from build123d import *

# Parameters (mm, degrees)
SKETCH_1_W          = 30
SKETCH_1_H          = 65
EXTRUDE_1_DEPTH     = 3
SKETCH_2_R          = 1.505
CUT_EXTRUDE_1_DEPTH = 3
FILLET_1_R          = 2
SKETCH_3_W          = 13
SKETCH_3_H          = 48
CUT_EXTRUDE_2_DEPTH = 10
FILLET_2_R          = 2


with BuildPart() as part:
    # 草图1 → 凸台-拉伸1 (new body)
    with BuildSketch(Plane.XY):
        Rectangle(SKETCH_1_W, SKETCH_1_H)
    extrude(amount=EXTRUDE_1_DEPTH)

    # 草图2 → 切除-拉伸1 (cut)
    with BuildSketch(Plane.XY.offset(3)):
        with Locations((-11, 28.5)):
            Circle(SKETCH_2_R)
        with Locations((11, 28.5)):
            Circle(SKETCH_2_R)
        with Locations((-11, 6.5)):
            Circle(SKETCH_2_R)
        with Locations((11, 6.5)):
            Circle(SKETCH_2_R)
    cut_extrude_1 = extrude(amount=-CUT_EXTRUDE_1_DEPTH, mode=Mode.SUBTRACT)

    # 镜向1: 切除-拉伸1 across plane
    add(cut_extrude_1.mirror(Plane.ZX), mode=Mode.SUBTRACT)

    # 圆角1
    fillet_1_edges = [part.edges().sort_by_distance(p)[0] for p in [
        (15, -32.5, 1.5),
        (-15, -32.5, 1.5),
        (-15, 32.5, 1.5),
        (15, 32.5, 1.5),
    ]]
    fillet(fillet_1_edges, radius=FILLET_1_R)

    # 草图3 → 切除-拉伸2 (cut)
    with BuildSketch(Plane.XY.offset(3)):
        Rectangle(SKETCH_3_W, SKETCH_3_H)
    extrude(amount=-CUT_EXTRUDE_2_DEPTH, mode=Mode.SUBTRACT)

    # 圆角2
    fillet_2_edges = [part.edges().sort_by_distance(p)[0] for p in [
        (6.5, 24, 1.5),
        (6.5, -24, 1.5),
        (-6.5, -24, 1.5),
        (-6.5, 24, 1.5),
    ]]
    fillet(fillet_2_edges, radius=FILLET_2_R)


solid = part.part
Design review of the part built by this model. Coordinates are the model's own, in mm. A direction names the side the tool comes from. Give positions to 0.01 mm unless a question says otherwise; leave off trailing zeros. Order: outer loops, then holes, each group sorted by start corner. A loop starts at its lowest first (then second) coordinate and runs counter-clockwise, first axis right, second up. Notation, with made-up numbers: (63, 44.25) - (112, 44.25) arc R15 ccw to (112, 64.25) - close; hole circle Ø9 at (21.5, 49.25). An arc over 180 degrees is marked (long way). Write item = value, one per line. Start each with the question number.
Q1. To check wall thickness, follow L1, parallel to Y at x = 11, z = 1.7 (3 decimals); L2, parallel to X at y = 1.5, z = 0.6; L3, parallel to Y at x = 3.75, z = 2.8. State the ranges of each line that lie inside material, in increasing order. Write a range as from..to.
Q2. We need section B-B on y = -2.5. State the section outline as (x, z) points.
Q3. Mouldability with a two-part tool opening along Y and no side actions: class faces 1 (the face through (-7, 0, 3)), 2 (the face through (-6.5, 0, 2)), 3 (the face through (-14.43, -31.9, 1.52)) as released by +Y, released by -Y, zero draft, split by the parting line, or undercut.
Q4. We need section A-A on y = 6.5. State the section outline as (x, z) points (3 decimals).
Q5. Tool access review of faces 4 (the face through (-14.43, 31.9, 1.52)), 5 (the face through (6.5, 0, 2)): name each direction out of +Z, -Z, +X, -X, +Y, -Y from which nothing blocks a thin tool from reaching the whole face with its end or side.
Q6. We need section D-D on x = 3. State the section outline as (y, z) points.
Q7. Clearance check with a flat-ended pin moving along its axis: pin 1 Ø4 at (x, y) = (-4, 16) entering from -Z. State where the tip first meets the part, or that it passes through.
Q8. We need section C-C on z = 2. State how many separate pieces and enclosed holes the cut face has, plus the area to 3 significant figures.
Working result:
q1.L1 = -32.5..-30.005, -26.995..-8.005, -4.995..4.995, 8.005..26.995, 30.005..32.5
q1.L2 = -15..-6.5, 6.5..15
q1.L3 = -32.5..-24, 24..32.5
q2.outline = (-15, 0) - (-6.5, 0) - (-6.5, 3) - (-15, 3) - close; (6.5, 0) - (15, 0) - (15, 3) - (6.5, 3) - close
q3.face_1 = zero draft
q3.face_2 = undercut
q3.face_3 = released by -Y
q4.outline = (-15, 0) - (-12.505, 0) - (-12.505, 3) - (-15, 3) - close; (-9.495, 0) - (-6.5, 0) - (-6.5, 3) - (-9.495, 3) - close; (6.5, 0) - (9.495, 0) - (9.495, 3) - (6.5, 3) - close; (12.505, 0) - (15, 0) - (15, 3) - (12.505, 3) - close
q5.face_4 = +Z, -Z, -X, +Y
q5.face_5 = +Z, -Z
q6.outline = (-32.5, 0) - (-24, 0) - (-24, 3) - (-32.5, 3) - close; (24, 0) - (32.5, 0) - (32.5, 3) - (24, 3) - close
q7.pin_1 = through
q8.separate_pieces = 1
q8.enclosed_holes = 9
q8.area = 1,270 mm²
